```python
from build123d import *

# Parameters (mm, degrees)
F0_R     = 5
F1_DEPTH = 15
F2_W     = 30
F2_H     = 30
F3_DEPTH = 5
F4_W     = 30
F4_H     = 15
F5_DEPTH = 5
F6_R     = 10
F7_DEPTH = 15


with BuildPart() as f1:
    # F0 (on Top) → F1 (new body)
    with BuildSketch(Plane.XY):
        Polygon((-135, 0), (-135, -35), (15, -60), (15, 0), (15, 60), (-135, 35), align=None)
        with Locations((0, -40)):
            Circle(F0_R, mode=Mode.SUBTRACT)
        with Locations((0, 40)):
            Circle(F0_R, mode=Mode.SUBTRACT)
    extrude(amount=F1_DEPTH)

    # F2 (on face) → F3 (join)
    with BuildSketch(Plane.XY.offset(15)):
        with Locations((-120, 0)):
            Rectangle(F2_W, F2_H)
    extrude(amount=F3_DEPTH)

    # F4 (on face) → F5 (cut)
    with BuildSketch(Plane.XY.offset(20)):
        with Locations((-120, 0)):
            Rectangle(F4_W, F4_H)
    extrude(amount=-F5_DEPTH, mode=Mode.SUBTRACT)

    # F6 (on face) → F7 (cut)
    with BuildSketch(Plane.XY.offset(15)):
        with Locations((-24.507769, 0)):
            Circle(F6_R)
    extrude(amount=-F7_DEPTH, mode=Mode.SUBTRACT)


solid = f1.part
```
The listing builds one solid part. Answer for the finished solid, in the listing's coordinates (mm). A direction names the side the tool comes from. Round coordinates to 2 decimals unless told otherwise and drop trailing zeros. Loops run counter-clockwise (first coordinate to the right, second up) from the corner with the lowest first, then second, coordinate; pieces in that order, holes last.
Q1. For a pull along X with two mould halves and no side action, classify faces 1 (the face through (-61.05, -47.325, 7.395)), 2 (the face through (-44, 1, 15)), 3 (the face through (-32.443, -6.085, 7.605)) as released by +X, released by -X, zero draft, split by the parting line, or undercut.
Q2. Section B-B, the plane z = 17.25 is taken. Determine the outline of the cut face in (x, y).
Q3. Given pin 1 Ø4 at (x, z) = (-115, 16.5) entering from +Y; pin 2 Ø8 at (x, z) = (-30.5, 10.5) entering from -Y; pin 3 Ø2.5 at (x, z) = (-115, 17) entering from -Y; pin 4 Ø1.5 at (x, z) = (-68, 16.5) entering from +Y, each flat-ended and moving along its own axis, determine where each tip first touches the part or whether it passes through.
Q4. Section C-C, the plane y = 0 is taken. Determine the outline of the cut face in (x, z).
Q5. Section A-A, the plane x = 0 is taken. Determine the outline of the cut face in (y, z).
Q6. Which of the six approach directions +Z, -Z, +X, -X, +Y, -Y give full straight-line access (tool end or side, diameter ignored) to faces 4 (the face through (-61, 1, 0)), 5 (the face through (-120, 15, 17)), 6 (the face through (-120, -15, 17)), 7 (the face through (-120, 7.5, 18)), 8 (the face through (-105, 11, 17))?
Q7. Section D-D, the plane z = 9.5 is taken. Determine the outline of the cut face in (x, y), then the cut area to 3 significant figures.
Q8. Find the intervals of material crossed by line 1 (Y direction, x = -108.5, z = 15.5); line 2 (Y direction, x = 0, z = 8); line 3 (X direction, y = -9, z = 6), in increasing order.
Completed:
1. face 1: released by -X
1. face 2: zero draft
1. face 3: undercut
2. outline: (-135, -15) - (-105, -15) - (-105, -7.5) - (-135, -7.5) - close; (-135, 7.5) - (-105, 7.5) - (-105, 15) - (-135, 15) - close
3. pin 1: stops at y = 38.55
3. pin 2: stops at y = -53.08
3. pin 3: stops at y = -15
3. pin 4: passes through
4. outline: (-135, 0) - (-34.51, 0) - (-34.51, 15) - (-135, 15) - close; (-14.51, 0) - (15, 0) - (15, 15) - (-14.51, 15) - close
5. outline: (-57.5, 0) - (-45, 0) - (-45, 15) - (-57.5, 15) - close; (-35, 0) - (35, 0) - (35, 15) - (-35, 15) - close; (45, 0) - (57.5, 0) - (57.5, 15) - (45, 15) - close
6. face 4: -Z, +X, -X, +Y, -Y
6. face 5: +Z, +X, -X, +Y
6. face 6: +Z, +X, -X, -Y
6. face 7: +Z, +X, -X
6. face 8: +Z, +X, +Y, -Y
7. outline: (-135, -35) - (15, -60) - (15, 60) - (-135, 35) - close; hole circle Ø20 at (-24.51, 0); hole circle Ø10 at (0, -40); hole circle Ø10 at (0, 40)
7. area: 13,800 mm2
8. line 1: y = -15 to -7.5, 7.5 to 15
8. line 2: y = -57.5 to -45, -35 to 35, 45 to 57.5
8. line 3: x = -135 to -28.87, -20.15 to 15
